```python
from build123d import *

# Parameters (mm, degrees)
SKETCH1_W           = 10.16
SKETCH1_H           = 29.21
SKETCH1_R           = 2.032
SKETCH1_R_2         = 4.1275
BOSS_EXTRUDE1_DEPTH = 12.7
SKETCH1_3_R         = 2.032
CUT_EXTRUDE2_DEPTH  = 21.010058096
CUT_EXTRUDE3_START  = 2.54
SKETCH1_4_R         = 4.1275
SKETCH1_4_R_2       = 2.032
CUT_EXTRUDE3_DEPTH  = 10.16
SKETCH2_R           = 4.05
CUT_EXTRUDE1_DEPTH  = 3.81
SKETCH3_R           = 2.54
CUT_EXTRUDE4_DEPTH  = 22.859131445
CHAMFER1_SIZE       = 8.89
FILLET1_R           = 6.35
FILLET2_R           = 6.35
CHAMFER2_SIZE       = 0.635


# Some blends are built 0.0001 mm under size
with BuildPart() as part:
    # Sketch1 → Boss-Extrude1 (new body)
    # profile 1 of 5: a face of its own
    with BuildSketch(Plane(origin=(0, 0, 0), x_dir=(1, 0, 0), z_dir=(0, 1, 0))):
        Rectangle(SKETCH1_W, SKETCH1_H)
        with Locations((0, -8.89)):
            Circle(SKETCH1_R, mode=Mode.SUBTRACT)
        with Locations((0, 1.27)):
            Circle(SKETCH1_R, mode=Mode.SUBTRACT)
    # profile 2 of 5: a face of its own
    with BuildSketch(Plane(origin=(0, 0, 0), x_dir=(1, 0, 0), z_dir=(0, 1, 0))):
        with Locations((0, 1.27)):
            Circle(SKETCH1_R_2)
        with Locations((0, 1.27)):
            Circle(SKETCH1_R, mode=Mode.SUBTRACT)
    # profile 3 of 5: a face of its own
    with BuildSketch(Plane(origin=(0, 0, 0), x_dir=(1, 0, 0), z_dir=(0, 1, 0))):
        with Locations((0, 1.27)):
            Circle(SKETCH1_R)
    # profile 4 of 5: a face of its own
    with BuildSketch(Plane(origin=(0, 0, 0), x_dir=(1, 0, 0), z_dir=(0, 1, 0))):
        with Locations((0, -8.89)):
            Circle(SKETCH1_R_2)
        with Locations((0, -8.89)):
            Circle(SKETCH1_R, mode=Mode.SUBTRACT)
    # profile 5 of 5: a face of its own
    with BuildSketch(Plane(origin=(0, 0, 0), x_dir=(1, 0, 0), z_dir=(0, 1, 0))):
        with Locations((0, -8.89)):
            Circle(SKETCH1_R)
    extrude(amount=BOSS_EXTRUDE1_DEPTH)

    # Sketch1<3> → Cut-Extrude2 (cut, through all)
    with BuildSketch(Plane(origin=(0, 0, 0), x_dir=(1, 0, 0), z_dir=(0, 1, 0))):
        with Locations(Location((0, 1.27, 0), (0, 0, 270))):
            Circle(SKETCH1_3_R)
        with Locations(Location((0, -8.89, 0), (0, 0, 270))):
            Circle(SKETCH1_3_R)
    extrude(amount=CUT_EXTRUDE2_DEPTH, mode=Mode.SUBTRACT)

    # Sketch1<4> → Cut-Extrude3 (cut)
    # profile 1 of 2: a face of its own
    with BuildSketch(Plane(origin=(0, 0, 0), x_dir=(1, 0, 0), z_dir=(0, 1, 0)).offset(CUT_EXTRUDE3_START)):
        with Locations(Location((0, -8.89, 0), (0, 0, 270))):
            Circle(SKETCH1_4_R)
        with Locations(Location((0, -8.89, 0), (0, 0, 270))):
            Circle(SKETCH1_4_R_2, mode=Mode.SUBTRACT)
    # profile 2 of 2: a face of its own
    with BuildSketch(Plane(origin=(0, 0, 0), x_dir=(1, 0, 0), z_dir=(0, 1, 0)).offset(CUT_EXTRUDE3_START)):
        with Locations(Location((0, 1.27, 0), (0, 0, 270))):
            Circle(SKETCH1_4_R)
        with Locations(Location((0, 1.27, 0), (0, 0, 270))):
            Circle(SKETCH1_4_R_2, mode=Mode.SUBTRACT)
    extrude(amount=CUT_EXTRUDE3_DEPTH, mode=Mode.SUBTRACT)

    # Sketch2 → Cut-Extrude1 (cut)
    with BuildSketch(Plane.ZY.offset(5.08)):
        with Locations((-8.255, 6.35)):
            Circle(SKETCH2_R)
    extrude(amount=-CUT_EXTRUDE1_DEPTH, mode=Mode.SUBTRACT)

    # Sketch3 → Cut-Extrude4 (cut, through all)
    with BuildSketch(Plane.ZY.offset(5.08)):
        with Locations((-8.255, 6.35)):
            Circle(SKETCH3_R)
    extrude(amount=-CUT_EXTRUDE4_DEPTH, mode=Mode.SUBTRACT)

    # Chamfer1
    # the kernel refuses this chamfer: 8.89 mm, written as the material it takes off along each edge
    with BuildSketch(Plane(origin=(-27.942261763, 12.7, 14.605), x_dir=(0, -0.9996219169112966, 0.027495876610586317), z_dir=(1, 0, 0))) as chamfer1_piece_1:
        Polygon((CHAMFER1_SIZE * 0.999621916911, CHAMFER1_SIZE * 0.0274958766106), (-CHAMFER1_SIZE * 0.0274958766106, CHAMFER1_SIZE * 0.999621916911), (0, 0), align=None)
    extrude(amount=55.884523526, mode=Mode.SUBTRACT)

    # Fillet1
    # the kernel refuses this fillet: 6.35 mm, written as the material it takes off along each edge
    with BuildSketch(Plane(origin=(-11.655640303, 3.81, 14.605), x_dir=(0, -1, 0), z_dir=(1, 0, 0))) as fillet1_piece_1:
        with BuildLine():
            CenterArc((FILLET1_R * 0.414213562373, FILLET1_R), FILLET1_R, 225, 45)
            Line((-FILLET1_R * 0.292893218814, FILLET1_R * 0.292893218814), (0, 0))
            Line((0, 0), (FILLET1_R * 0.414213562373, 0))
        make_face()
    extrude(amount=23.311280605, mode=Mode.SUBTRACT)
    with BuildSketch(Plane(origin=(-11.655640303, 12.7, 5.715), x_dir=(0, -0.7071067811862649, 0.7071067811868301), z_dir=(1, 0, 0)), Plane(origin=(-3.938287226, 12.7, 5.715), x_dir=(0, -0.7071067811862649, 0.7071067811868301), z_dir=(1, 0, 0))) as fillet1_piece_2:
        with BuildLine():
            CenterArc((FILLET1_R * 0.414213562373, FILLET1_R), FILLET1_R, 225, 45)
            Line((-FILLET1_R * 0.292893218813, FILLET1_R * 0.292893218813), (0, 0))
            Line((0, 0), (FILLET1_R * 0.414213562373, 0))
        make_face()
    extrude(amount=15.593927529, mode=Mode.SUBTRACT)

    # Fillet2
    fillet2_edges = [part.edges().sort_by_distance(p)[0] for p in [
        (0, 12.7, -14.605),
        (0, 0, -14.605),
    ]]
    fillet(fillet2_edges, radius=FILLET2_R - 0.0001)  # a hair under: the kernel refuses the full size

    # Chamfer2
    # the kernel refuses this chamfer: 0.635 mm, written as the material it takes off along each edge
    with BuildSketch(Plane(origin=(0, 0, -1.27), x_dir=(0, 0, 1), z_dir=(-1, 0, 0))) as chamfer2_piece_1:
        Polygon((2.032 + CHAMFER2_SIZE, 0), (2.032, CHAMFER2_SIZE), (2.032, 0), align=None)
    revolve(axis=Axis((0, 0, -1.27), (0, 1, 0)), mode=Mode.SUBTRACT)
    with BuildSketch(Plane(origin=(0, 0, 8.89), x_dir=(0, 0, 1), z_dir=(-1, 0, 0))) as chamfer2_piece_2:
        Polygon((2.032 + CHAMFER2_SIZE, 0), (2.032, CHAMFER2_SIZE), (2.032, 0), align=None)
    revolve(axis=Axis((0, 0, 8.89), (0, 1, 0)), mode=Mode.SUBTRACT)
    with BuildSketch(Plane(origin=(0, 2.54, 8.89), x_dir=(0, 0, 1), z_dir=(-1, 0, 0))) as chamfer2_piece_3:
        Polygon((2.032, -CHAMFER2_SIZE), (2.032 + CHAMFER2_SIZE, 0), (2.032, 0), align=None)
    revolve(axis=Axis((0, 2.54, 8.89), (0, 1, 0)), mode=Mode.SUBTRACT)
    with BuildSketch(Plane(origin=(0, 2.54, -1.27), x_dir=(0, 0, 1), z_dir=(-1, 0, 0))) as chamfer2_piece_4:
        Polygon((2.032, -CHAMFER2_SIZE), (2.032 + CHAMFER2_SIZE, 0), (2.032, 0), align=None)
    revolve(axis=Axis((0, 2.54, -1.27), (0, 1, 0)), mode=Mode.SUBTRACT)
    with BuildSketch(Plane(origin=(-5.08, 6.35, -8.255), x_dir=(0, 0, 1), z_dir=(0, -1, 0))) as chamfer2_piece_5:
        Polygon((4.05 + CHAMFER2_SIZE, 0), (4.05, -CHAMFER2_SIZE), (4.05, 0), align=None)
    revolve(axis=Axis((-5.08, 6.35, -8.255), (-1, 0, 0)), mode=Mode.SUBTRACT)
    with BuildSketch(Plane(origin=(-1.27, 6.35, -8.255), x_dir=(0, 0, 1), z_dir=(0, -1, 0))) as chamfer2_piece_6:
        Polygon((2.54 + CHAMFER2_SIZE, 0), (2.54, -CHAMFER2_SIZE), (2.54, 0), align=None)
    revolve(axis=Axis((-1.27, 6.35, -8.255), (-1, 0, 0)), mode=Mode.SUBTRACT)
    with BuildSketch(Plane(origin=(5.08, 6.35, -8.255), x_dir=(0, 0, 1), z_dir=(0, -1, 0))) as chamfer2_piece_7:
        Polygon((2.54 + CHAMFER2_SIZE, 0), (2.54, CHAMFER2_SIZE), (2.54, 0), align=None)
    revolve(axis=Axis((5.08, 6.35, -8.255), (-1, 0, 0)), mode=Mode.SUBTRACT)
    with BuildSketch(Plane(origin=(-5.08, 0, -8.2551), x_dir=(-0.027495876610585925, 0.9996219169112968, 0), z_dir=(0, 0, 1))) as chamfer2_piece_8:
        Polygon((CHAMFER2_SIZE * 0.999621916911, -CHAMFER2_SIZE * 0.0274958766106), (-CHAMFER2_SIZE * 0.0274958766106, -CHAMFER2_SIZE * 0.999621916911), (0, 0), align=None)
    extrude(amount=24.493118697, mode=Mode.SUBTRACT)
    with BuildSketch(Plane(origin=(5.08, -1.633018697, 14.605), x_dir=(-0.9996219169112966, 0, 0.027495876610587302), z_dir=(0, 1, 0)), Plane(origin=(-5.08, -1.633018697, 14.605), x_dir=(-0.027495876610585834, 0, -0.9996219169112968), z_dir=(0, 1, 0))) as chamfer2_piece_9:
        Polygon((CHAMFER2_SIZE * 0.999621916911, -CHAMFER2_SIZE * 0.0274958766106), (-CHAMFER2_SIZE * 0.0274958766106, -CHAMFER2_SIZE * 0.999621916911), (0, 0), align=None)
    extrude(amount=2.812762576, mode=Mode.SUBTRACT)
    with BuildSketch(Plane(origin=(-5.08, 10.840128061, 7.574871939), x_dir=(-0.027495876610587233, -0.706839436070956, -0.7068394360703909), z_dir=(0, -0.7071067811862648, 0.7071067811868302)), Plane(origin=(5.08, 5.669871939, 12.745128061), x_dir=(0.02749587661058726, -0.7068394360709561, -0.7068394360703909), z_dir=(0, 0.7071067811862648, -0.7071067811868302))) as chamfer2_piece_10:
        Polygon((CHAMFER2_SIZE * 0.999621916911, CHAMFER2_SIZE * 0.0274958766106), (-CHAMFER2_SIZE * 0.0274958766106, CHAMFER2_SIZE * 0.999621916911), (0, 0), align=None)
    extrude(amount=7.311846327, mode=Mode.SUBTRACT)
    with BuildSketch(Plane(origin=(-5.08, 12.7, -8.2551), x_dir=(-0.02749587661058591, -0.9996219169112968, 0), z_dir=(0, 0, 1))) as chamfer2_piece_11:
        Polygon((CHAMFER2_SIZE * 0.999621916911, CHAMFER2_SIZE * 0.0274958766106), (-CHAMFER2_SIZE * 0.0274958766106, CHAMFER2_SIZE * 0.999621916911), (0, 0), align=None)
    extrude(amount=11.339843879, mode=Mode.SUBTRACT)
    with BuildSketch(Plane(origin=(-5.08, 6.35, 3.084743879), x_dir=(0, 0.7071067811870476, 0.7071067811860474), z_dir=(0, -0.7071067811860474, 0.7071067811870476))) as chamfer2_piece_12:
        Polygon((6.35 - CHAMFER2_SIZE, 0), (6.35, -CHAMFER2_SIZE), (6.35, 0), align=None)
    revolve(axis=Axis((-5.08, 6.35, 3.084743879), (-1, 0, 0)), revolution_arc=45, mode=Mode.SUBTRACT)
    with BuildSketch(Plane(origin=(5.08, 0, 16.238018697), x_dir=(-0.9996219169112966, -0.0274958766105864, 0), z_dir=(0, 0, -1))) as chamfer2_piece_13:
        Polygon((CHAMFER2_SIZE * 0.999621916911, CHAMFER2_SIZE * 0.0274958766106), (-CHAMFER2_SIZE * 0.0274958766106, CHAMFER2_SIZE * 0.999621916911), (0, 0), align=None)
    extrude(amount=24.493118697, mode=Mode.SUBTRACT)
    with BuildSketch(Plane(origin=(-5.08, 1.179743879, 8.255), x_dir=(0, 0, 1), z_dir=(0, -1, 0))) as chamfer2_piece_14:
        Polygon((6.35 - CHAMFER2_SIZE, 0), (6.35, -CHAMFER2_SIZE), (6.35, 0), align=None)
    revolve(axis=Axis((-5.08, 1.179743879, 8.255), (-1, 0, 0)), revolution_arc=45, mode=Mode.SUBTRACT)
    with BuildSketch(Plane(origin=(5.08, 12.7, 3.084743879), x_dir=(-0.9996219169112966, 0.027495876610587302, 0), z_dir=(0, 0, -1))) as chamfer2_piece_15:
        Polygon((CHAMFER2_SIZE * 0.999621916911, -CHAMFER2_SIZE * 0.0274958766106), (-CHAMFER2_SIZE * 0.0274958766106, -CHAMFER2_SIZE * 0.999621916911), (0, 0), align=None)
    extrude(amount=11.339843879, mode=Mode.SUBTRACT)
    with BuildSketch(Plane(origin=(5.08, 6.35, 3.084743879), x_dir=(0, 0.7071067811870476, 0.7071067811860474), z_dir=(0, -0.7071067811860474, 0.7071067811870476))) as chamfer2_piece_16:
        Polygon((6.35, CHAMFER2_SIZE), (6.35 - CHAMFER2_SIZE, 0), (6.35, 0), align=None)
    revolve(axis=Axis((5.08, 6.35, 3.084743879), (-1, 0, 0)), revolution_arc=45, mode=Mode.SUBTRACT)
    with BuildSketch(Plane(origin=(5.08, 1.179743879, 8.255), x_dir=(0, 0, 1), z_dir=(0, -1, 0))) as chamfer2_piece_17:
        Polygon((6.35, CHAMFER2_SIZE), (6.35 - CHAMFER2_SIZE, 0), (6.35, 0), align=None)
    revolve(axis=Axis((5.08, 1.179743879, 8.255), (-1, 0, 0)), revolution_arc=45, mode=Mode.SUBTRACT)
    with BuildSketch(Plane(origin=(5.08, 6.3501, -8.2551), x_dir=(0, 0, -1), z_dir=(0, -1, 0))) as chamfer2_piece_18:
        Polygon((6.3499, -CHAMFER2_SIZE), (6.3499 - CHAMFER2_SIZE, 0), (6.3499, 0), align=None)
    revolve(axis=Axis((5.08, 6.3501, -8.2551), (1, 0, 0)), revolution_arc=90, mode=Mode.SUBTRACT)
    with BuildSketch(Plane(origin=(5.08, 6.3499, -8.2551), x_dir=(0, 0, -1), z_dir=(0, 1, 0))) as chamfer2_piece_19:
        Polygon((6.3499, CHAMFER2_SIZE), (6.3499 - CHAMFER2_SIZE, 0), (6.3499, 0), align=None)
    revolve(axis=Axis((5.08, 6.3499, -8.2551), (-1, 0, 0)), revolution_arc=90, mode=Mode.SUBTRACT)
    with BuildSketch(Plane(origin=(-5.08, 6.3501, -8.2551), x_dir=(0, 0, -1), z_dir=(0, -1, 0))) as chamfer2_piece_20:
        Polygon((6.3499 - CHAMFER2_SIZE, 0), (6.3499, CHAMFER2_SIZE), (6.3499, 0), align=None)
    revolve(axis=Axis((-5.08, 6.3501, -8.2551), (1, 0, 0)), revolution_arc=90, mode=Mode.SUBTRACT)
    with BuildSketch(Plane(origin=(-5.08, 6.3499, -8.2551), x_dir=(0, 0, -1), z_dir=(0, 1, 0))) as chamfer2_piece_21:
        Polygon((6.3499 - CHAMFER2_SIZE, 0), (6.3499, -CHAMFER2_SIZE), (6.3499, 0), align=None)
    revolve(axis=Axis((-5.08, 6.3499, -8.2551), (-1, 0, 0)), revolution_arc=90, mode=Mode.SUBTRACT)
    with BuildSketch(Plane(origin=(-5.08, 6.3499, -14.605), x_dir=(-0.02749587661058591, 0, 0.9996219169112968), z_dir=(0, 1, 0)), Plane(origin=(5.08, 6.3499, -14.605), x_dir=(-0.9996219169112966, 0, -0.027495876610587302), z_dir=(0, 1, 0))) as chamfer2_piece_22:
        Polygon((CHAMFER2_SIZE * 0.999621916911, CHAMFER2_SIZE * 0.0274958766106), (-CHAMFER2_SIZE * 0.0274958766106, CHAMFER2_SIZE * 0.999621916911), (0, 0), align=None)
    extrude(amount=0.0002, mode=Mode.SUBTRACT)


solid = part.part
```
Work out the finished part from the listing and answer in its coordinate system (mm). A direction names the side the tool comes from. Round coordinates to 2 decimals unless told otherwise and drop trailing zeros. Write each question's results on one line, items separated by ' | '.
1) For a pull along X with two mould halves and no side action, classify faces 4 (the cylindrical face through (0.062, 10.889, -12.696)), 5 (the conical face through (-4.83, 11.85, 5.4)), 6 (the flat face through (-3, 2.54, -1)) as +X half, -X half, draft (parallel to the pull), parting line (faces both ways), or undercut.
Findings:
face 4: draft | face 5: -X half | face 6: undercut
2) Flat-ended cylindrical pins translate along their axes: pin 1 (3 mm diameter, centred on x = 3.5, y = 8.5, fed in from +Z) (3 decimals); pin 2 (2.5 mm diameter, centred on x = -1.5, z = 8, fed in from +Y); pin 3 (2 mm diameter, centred on y = 5, z = -9.5, fed in from -X). Find the tip coordinate at first contact, or state that the pin passes through.
Findings:
pin 1: stops at z = 11.415 | pin 2: stops at y = 2.54 | pin 3: stops at x = -0.93
3) The part is cut by section B-B (x = 0). State how many separate pieces and enclosed holes the cut face has, and give its area (3 significant figures).
Findings:
separate pieces: 3 | enclosed holes: 1 | area: 130 mm²
4) Consider line 1 along X through (y, z) = (1.6, 8.89); line 2 along X through (y, z) = (5, 9); line 3 along Z through (x, y) = (-4.5, 7.25). Determine where each line is inside the solid, lowest interval first. Write a range as [from, to].
Findings:
line 1: x = [-5.08, -2.03], [2.03, 5.08] | line 2: x = [-5.08, -4.13], [4.13, 5.08] | line 3: z = [-14.49, -12.26], [-4.25, 11.09]
5) Which of the six approach directions +Z, -Z, +X, -X, +Y, -Y give full straight-line access (tool end or side, diameter ignored) to faces 1 (the flat face through (4.767, 7.991, 9.969)), 2 (the cylindrical face through (0.181, 6.334, 4.766)), 3 (the cylindrical face through (-2.88, 6.53, -12.3))?
Findings:
face 1: +Z, +X, +Y | face 2: +Y | face 3: -X
